Build history of the part. All positions in model axes, mm. Face numbers are marked on the shaded views. A direction names the side the tool comes from. Give positions to 0.01 mm unless a question says otherwise; leave off trailing zeros. Write each loop counter-clockwise with the first axis right and the second up, starting at its lowest first coordinate (ties: lowest second). Pieces come first, ordered by that corner, then holes. Notation, with made-up numbers: (-1, 42) -> (18, 42) arc R23 ccw to (18, 61) -> close; hole circle Ø7 at (-1, 53.5). An arc over 180 degrees is marked (long way). Put each result on its own line as item: value. Start each with the question number.
Item 1: Drill centre lines: line 1 along Z through (x, y) = (-10.5, 0.5); line 2 along X through (y, z) = (3.5, -5); line 3 along Z through (x, y) = (-3.5, 5.5). Where is each one in solid material? Low to high.
Item 2: Slice it at D-D, the plane y = 2.5. List the corners of the cut face in (x, z), plus the area to 3 significant figures.
Item 3: Slice it at C-C, the plane x = 3.25. List the corners of the cut face in (y, z).
Item 4: Tool access for the marked faces 1, 2 and 3: list every direction of +Z, -Z, +X, -X, +Y, -Y with a clear straight run to the whole face (end or side of a thin tool).
Item 5: Flat gauge pins, fed straight in: pin 1 Ø3 at (y, z) = (5, -3.5) entering from +X; pin 2 Ø2.5 at (x, z) = (-10.5, 9.931) entering from +Y; pin 3 Ø2 at (x, y) = (-0.5, 3) entering from +Z. Where does each tip first touch, or does it go through?
Item 6: Slice it at A-A, the plane x = 10.5. List the corners of the cut face in (y, z).
Item 7: Slice it at B-B, the plane z = 6.5. List the corners of the cut face in (x, y), plus the area to 3 significant figures.
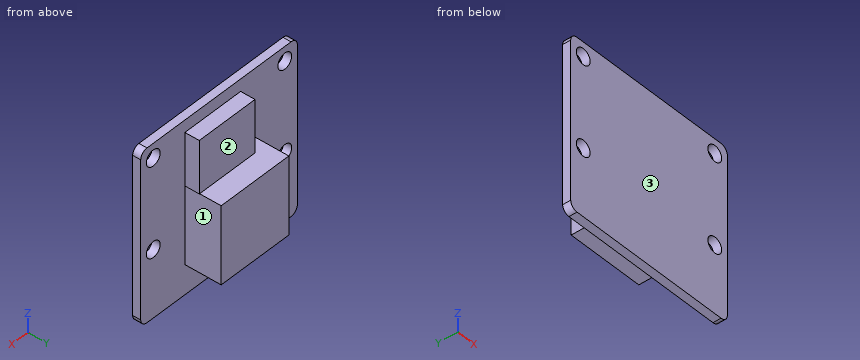
```python
from build123d import *

# Parameters (mm, degrees)
SKETCH1_W           = 25
SKETCH1_H           = 23.862
BOSS_EXTRUDE1_DEPTH = 1.12
FILLET1_R           = 1
SKETCH2_R           = 1.1
CUT_EXTRUDE1_DEPTH  = 2
SKETCH3_W           = 10.8
SKETCH3_H           = 10.8
BOSS_EXTRUDE2_DEPTH = 5
SKETCH4_W           = 8.9
SKETCH4_H           = 7.3
BOSS_EXTRUDE3_DEPTH = 2


with BuildPart() as part:
    # Sketch1 → Boss-Extrude1 (new body)
    with BuildSketch(Plane(origin=(0, 0, 0), x_dir=(1, 0, 0), z_dir=(0, 1, 0))):
        Rectangle(SKETCH1_W, SKETCH1_H)
    extrude(amount=BOSS_EXTRUDE1_DEPTH)

    # Fillet1
    fillet1_edges = [part.edges().sort_by_distance(p)[0] for p in [
        (-12.5, 0.56, -11.931),
        (12.5, 0.56, -11.931),
        (12.5, 0.56, 11.931),
        (-12.5, 0.56, 11.931),
    ]]
    fillet(fillet1_edges, radius=FILLET1_R)

    # Sketch2 → Cut-Extrude1 (cut)
    with BuildSketch(Plane(origin=(0, 1.12, 0), x_dir=(1, 0, 0), z_dir=(0, 1, 0))):
        with Locations((-10.5, 2.569)):
            Circle(SKETCH2_R)
        with Locations((10.5, 2.569)):
            Circle(SKETCH2_R)
        with Locations((-10.5, -9.931)):
            Circle(SKETCH2_R)
        with Locations((10.5, -9.931)):
            Circle(SKETCH2_R)
    extrude(amount=-CUT_EXTRUDE1_DEPTH, mode=Mode.SUBTRACT)

    # Sketch3 → Boss-Extrude2 (add)
    with BuildSketch(Plane(origin=(0, 1.12, 0), x_dir=(1, 0, 0), z_dir=(0, 1, 0))):
        with Locations((0, 2.469)):
            Rectangle(SKETCH3_W, SKETCH3_H)
    extrude(amount=BOSS_EXTRUDE2_DEPTH)

    # Sketch4 → Boss-Extrude3 (add)
    with BuildSketch(Plane(origin=(0, 1.12, 0), x_dir=(1, 0, 0), z_dir=(0, 1, 0))):
        with Locations((1, -6.581)):
            Rectangle(SKETCH4_W, SKETCH4_H)
    extrude(amount=BOSS_EXTRUDE3_DEPTH)


solid = part.part
```
Values follow:
1. line 1: -11.93 to -3.67, -1.47 to 8.83, 11.03 to 11.93
1. line 2: -5.4 to 5.4
1. line 3: -7.87 to 2.93
2. outline: (-5.4, -7.87) -> (5.4, -7.87) -> (5.4, 2.93) -> (5.45, 2.93) -> (5.45, 10.23) -> (-3.45, 10.23) -> (-3.45, 2.93) -> (-5.4, 2.93) -> close
2. area: 182 mm2
3. outline: (0, -11.93) -> (1.12, -11.93) -> (1.12, -7.87) -> (6.12, -7.87) -> (6.12, 2.93) -> (3.12, 2.93) -> (3.12, 10.23) -> (1.12, 10.23) -> (1.12, 11.93) -> (0, 11.93) -> close
4. face 1: -Z, +X, +Y
4. face 2: +Z, +X, -X, +Y
4. face 3: +Z, -Z, +X, -X, -Y
5. pin 1: x = 5.4
5. pin 2: y = 1.12
5. pin 3: z = 10.23
6. outline: (0, -11.93) -> (1.12, -11.93) -> (1.12, -3.67) -> (0, -3.67) -> close; (0, -1.47) -> (1.12, -1.47) -> (1.12, 8.83) -> (0, 8.83) -> close; (0, 11.03) -> (1.12, 11.03) -> (1.12, 11.93) -> (0, 11.93) -> close
7. outline: (-12.5, 0) -> (12.5, 0) -> (12.5, 1.12) -> (5.45, 1.12) -> (5.45, 3.12) -> (-3.45, 3.12) -> (-3.45, 1.12) -> (-12.5, 1.12) -> close
7. area: 45.8 mm2
